Build history of the part. All positions in model axes, mm. A direction names the side the tool comes from. Give positions to 0.01 mm unless a question says otherwise; leave off trailing zeros. Loops run counter-clockwise (first coordinate to the right, second up) from the corner with the lowest first, then second, coordinate; pieces in that order, holes last. Notation, with made-up numbers: M 86.25,29.5 L 143.25,29.5 A24 ccw 143.25,55.5 Z; hole C 40,51.25 d5. An arc over 180 degrees is marked long. Answer as a JSON object with one key per item and string values. Group by question number.
1. Drill centre lines: line 1 along Y through (x, z) = (0.6, -62.5); line 2 along Y through (x, z) = (1.25, -92); line 3 along Y through (x, z) = (4.15, -48). Where is each one in solid material? Low to high. Write a range as [from, to].
2. 3-axis set-ups, long thin cutter, end or side, ignore diameter. For faces 4 (the face through (2.5, 86, -54)), 5 (the face through (2, 45, -5)), 6 (the face through (2, 5, -54)), 7 (the face through (2, 25, -105)), 8 (the face through (2, 12, -107)): which of +Z, -Z, +X, -X, +Y, -Y reach the whole face in a straight line?
3. Slice it at A-A (x = 0.9). List the corners of the cut face in (y, z).
4. Mould opens along Z. For faces 1 (the face through (2, 45, -102)), 2 (the face through (0, 46, -53)), 3 (the face through (1, 87.5, -54)) say: released by +Z, released by -Z, zero draft, split by the parting line, or undercut.
5. Slice it at D-D (z = -94.5). List the corners of the cut face in (x, y).
6. Slice it at B-B (z = -70.5). List the corners of the cut face in (x, y).
7. Slice it at C-C (y = 37). List the corners of the cut face in (x, z).
8. Drop flat-ended pins along their axis: pin 1 Ø1.5 at (x, y) = (1.5, 58) entering from -Z; pin 2 Ø0.8 at (x, z) = (1, -49.5) entering from -Y; pin 3 Ø1.5 at (y, z) = (85.5, -61.5) entering from -X. Give the stop position or say it passes through.
from build123d import *

# Parameters (mm, degrees)
SKETCH1_W           = 107
SKETCH1_H           = 90
BOSS_EXTRUDE1_DEPTH = 5
SKETCH5_W           = 5
SKETCH5_H           = 40
SKETCH5_W_2         = 50
SKETCH5_H_2         = 5
CUT_EXTRUDE2_DEPTH  = 140.907112042
SKETCH6_W           = 102
SKETCH6_H           = 3
CUT_EXTRUDE3_DEPTH  = 2.5


with BuildPart() as part:
    # Sketch1 → Boss-Extrude1 (new body)
    with BuildSketch(Plane(origin=(0, 0, 0), x_dir=(0, 0, -1), z_dir=(1, 0, 0))):
        with Locations((53.5, 45)):
            Rectangle(SKETCH1_W, SKETCH1_H)
    extrude(amount=BOSS_EXTRUDE1_DEPTH)

    # Sketch5 → Cut-Extrude2 (cut, through all)
    with BuildSketch(Plane.ZY):
        with Locations((-104.5, 45)):
            Rectangle(SKETCH5_W, SKETCH5_H)
        with Locations((-2.5, 45)):
            Rectangle(SKETCH5_W, SKETCH5_H)
        with Locations((-53.5, 2.5)):
            Rectangle(SKETCH5_W_2, SKETCH5_H_2)
    extrude(amount=-CUT_EXTRUDE2_DEPTH, mode=Mode.SUBTRACT)

    # Sketch6 → Cut-Extrude3 (cut)
    with BuildSketch(Plane.ZY):
        with Locations((-53.5, 86)):
            Rectangle(SKETCH6_W, SKETCH6_H)
    extrude(amount=-CUT_EXTRUDE3_DEPTH, mode=Mode.SUBTRACT)


solid = part.part
Established:
{
 "1": {"line 1": "y = [5, 84.5], [87.5, 90]", "line 2": "y = [0, 84.5], [87.5, 90]", "line 3": "y = [5, 90]"},
 "2": {"face 4": "-X", "face 5": "+Z, +X, -X", "face 6": "+X, -X, -Y", "face 7": "-Z, +X, -X", "face 8": "-Z, +X, -X, +Y, -Y"},
 "3": {"outline": "M 0,-107 L 25,-107 L 25,-102 L 65,-102 L 65,-107 L 90,-107 L 90,0 L 65,0 L 65,-5 L 25,-5 L 25,0 L 0,0 L 0,-28.5 L 5,-28.5 L 5,-78.5 L 0,-78.5 Z; hole M 84.5,-104.5 L 87.5,-104.5 L 87.5,-2.5 L 84.5,-2.5 Z"},
 "4": {"face 1": "released by -Z", "face 2": "zero draft", "face 3": "undercut"},
 "5": {"outline": "M 0,0 L 5,0 L 5,90 L 0,90 L 0,87.5 L 2.5,87.5 L 2.5,84.5 L 0,84.5 Z"},
 "6": {"outline": "M 0,5 L 5,5 L 5,90 L 0,90 L 0,87.5 L 2.5,87.5 L 2.5,84.5 L 0,84.5 Z"},
 "7": {"outline": "M 0,-102 L 5,-102 L 5,-5 L 0,-5 Z"},
 "8": {"pin 1": "stops at z = -102", "pin 2": "stops at y = 5", "pin 3": "stops at x = 2.5"}
}
